from build123d import *

# Parameters (mm, degrees)
F0_W     = 28
F0_H     = 18
F1_DEPTH = 18
F2_R     = 4
F4_DEPTH = 18.001
F3_R     = 4
F5_DEPTH = 18.001
F6_R     = 1.25
F7_DEPTH = 28.001
F8_R     = 4


with BuildPart() as f1:
    # F0 (on Top) → F1 (new body)
    with BuildSketch(Plane.XY):
        Rectangle(F0_W, F0_H)
    extrude(amount=F1_DEPTH)

    # F2 (on face) → F4 (cut, through all)
    with BuildSketch(Plane.XY.offset(18)):
        with Locations((-5, 0)):
            Circle(F2_R)
    extrude(amount=-F4_DEPTH, mode=Mode.SUBTRACT)

    # F3 (on face) → F5 (cut, through all)
    with BuildSketch(Plane(origin=(0, 9, 0), x_dir=(-1, 0, 0), z_dir=(0, 1, 0))):
        with Locations((-5, 9)):
            Circle(F3_R)
    extrude(amount=-F5_DEPTH, mode=Mode.SUBTRACT)

    # F6 (on face) → F7 (cut, through all)
    with BuildSketch(Plane(origin=(-14, 0, 0), x_dir=(0, -1, 0), z_dir=(-1, 0, 0))):
        with Locations((0, 9)):
            Circle(F6_R)
    extrude(amount=-F7_DEPTH, mode=Mode.SUBTRACT)

    # F8
    f8_edges = [f1.edges().sort_by_distance(p)[0] for p in [
        (-14, -9, 9),
        (-14, 9, 9),
        (14, -9, 9),
        (14, 9, 9),
    ]]
    fillet(f8_edges, radius=F8_R)


solid = f1.part
Source: CAD feature listing. Evaluate the final solid. Frame: model axes, mm. Give positions to 0.01 mm unless a question says otherwise; leave off trailing zeros. Order: outer loops, then holes, each group sorted by start corner. A loop starts at its lowest first (then second) coordinate and runs counter-clockwise, first axis right, second up. Notation, with made-up numbers: (-35, -1.5) -> (6, -1.5) arc R20 cw to (6, 37.5) -> close; hole circle Ø9 at (5.5, 10.25). An arc over 180 degrees is marked (long way). Write item = value, one per line.
Q1. Cut plane D-D, the plane z = 9. Output: boundary loops of the cut face in (x, y).
Data:
outline = (-14, -5) arc R4 ccw to (-10, -9) -> (1, -9) -> (1, -1.25) -> (-1.2, -1.25) arc R4 cw to (-8.8, -1.25) -> (-14, -1.25) -> close; (-14, 1.25) -> (-8.8, 1.25) arc R4 cw to (-1.2, 1.25) -> (1, 1.25) -> (1, 9) -> (-10, 9) arc R4 ccw to (-14, 5) -> close; (9, -9) -> (10, -9) arc R4 ccw to (14, -5) -> (14, -1.25) -> (9, -1.25) -> close; (9, 1.25) -> (14, 1.25) -> (14, 5) arc R4 ccw to (10, 9) -> (9, 9) -> close
Q2. Cut plane C-C, the plane x = -5. Output: boundary loops of the cut face in (y, z).
Data:
outline = (-9, 0) -> (-4, 0) -> (-4, 18) -> (-9, 18) -> close; (4, 0) -> (9, 0) -> (9, 18) -> (4, 18) -> close
Q3. Cut plane A-A, the plane z = 12.25. Output: boundary loops of the cut face in (x, y), and give its area (3 significant figures).
Data:
outline = (-14, -5) arc R4 ccw to (-10, -9) -> (2.67, -9) -> (2.67, 9) -> (-10, 9) arc R4 ccw to (-14, 5) -> close; (7.33, -9) -> (10, -9) arc R4 ccw to (14, -5) -> (14, 5) arc R4 ccw to (10, 9) -> (7.33, 9) -> close; hole circle Ø8 at (-5, 0)
area = 356 mm^2
Q4. Pull-direction query (Y, two-part tool) for faces 1 (the face through (0, -9, 9)), 2 (the face through (11.36, 0.16, 10.24)), 3 (the face through (0, 0, 0)), 4 (the face through (-11.44, 0.16, 10.24)); classes: released by +Y, released by -Y, zero draft, split by the parting line, or undercut.
Data:
face_1 = released by -Y
face_2 = undercut
face_3 = zero draft
face_4 = undercut
Q5. Pin query (flat end, axial travel): pin 1 (4 mm diameter, centred on y = 0, z = 9, fed in from +X). Return the tip coordinate at first contact, or that it passes through.
Data:
pin_1 = 14
Q6. Material intervals for line 1 (Z direction, x = 11.35, y = 0); line 2 (X direction, y = 1.75, z = 6.5); line 3 (X direction, y = 0, z = 7.25), sorted ascending. Write a range as from..to.
Data:
line_1 = 0..7.75, 10.25..18
line_2 = -14..-8.6, -1.4..1.88, 8.12..14
line_3 = -14..-9, -1..1.4, 8.6..14
Q7. Cut plane B-B, the plane y = 2.75. Output: boundary loops of the cut face in (x, z).
Data:
outline = (-14, 0) -> (-7.9, 0) -> (-7.9, 18) -> (-14, 18) -> close; (-2.1, 0) -> (14, 0) -> (14, 18) -> (-2.1, 18) -> close; hole circle Ø8 at (5, 9)
